from build123d import *

# Parameters (mm, degrees)
SKETCH1_R           = 8
SKETCH1_R_2         = 5
SKETCH1_R_3         = 3.5
BOSS_EXTRUDE1_DEPTH = 48.5
BOSS_EXTRUDE2_START = 18
SKETCH3_R           = 3.5
BOSS_EXTRUDE2_DEPTH = 18
FILLET1_DEPTH       = 19
CUT_EXTRUDE1_START  = -30.5
CUT_EXTRUDE1_DEPTH  = 30.5
BOSS_EXTRUDE3_DEPTH = 9.5


with BuildPart() as part:
    # Sketch1 → Boss-Extrude1 (new body)
    # profile 1 of 4: a face of its own
    with BuildSketch(Plane.XY):
        with BuildLine():
            Line((15, -14), (17.94787914, -14))
            ThreePointArc((17.94787914, -14), (20, -13.638155725), (21.804604798, -12.596266659))
            Line((21.804604798, -12.596266659), (33.266394429, -2.978683207))
            ThreePointArc((33.266394429, -2.978683207), (35.857071693, -1.449912319), (38.688110115, -0.433068885))
            Line((38.688110115, -0.433068885), (56, 4))
            ThreePointArc((56, 4), (51, 9), (56, 14))
            Line((56, 14), (15, 14))
            Line((15, 14), (15, -14))
        make_face()
    # profile 2 of 4: a face of its own
    with BuildSketch(Plane.XY):
        with BuildLine():
            Line((-8, -14), (15, -14))
            Line((15, -14), (15, 14))
            Line((15, 14), (-4, 14))
            ThreePointArc((-4, 14), (-11.071067812, 11.071067812), (-14, 4))
            Line((-14, 4), (-14, -8))
            ThreePointArc((-14, -8), (-12.242640687, -12.242640687), (-8, -14))
        make_face()
        Circle(SKETCH1_R, mode=Mode.SUBTRACT)
    # profile 3 of 4: a face of its own
    with BuildSketch(Plane.XY):
        with Locations((56, 9)):
            Circle(SKETCH1_R_2)
        with Locations((56, 9)):
            Circle(SKETCH1_R_3, mode=Mode.SUBTRACT)
    # profile 4 of 4: a face of its own
    with BuildSketch(Plane.XY):
        with Locations((56, 9)):
            Circle(SKETCH1_R_3)
    extrude(amount=-BOSS_EXTRUDE1_DEPTH)

    # Sketch3 → Boss-Extrude2 (add)
    with BuildSketch(Plane.XY.offset(BOSS_EXTRUDE2_START)):
        with BuildLine():
            Line((38.688110115, -0.433068885), (56, 4))
            ThreePointArc((56, 4), (51, 9), (56, 14))
            Line((56, 14), (15, 14))
            Line((15, 14), (15, -14))
            Line((15, -14), (17.94787914, -14))
            ThreePointArc((17.94787914, -14), (20, -13.638155725), (21.804604798, -12.596266659))
            Line((21.804604798, -12.596266659), (33.266394429, -2.978683207))
            ThreePointArc((33.266394429, -2.978683207), (35.857071693, -1.449912319), (38.688110115, -0.433068885))
        make_face()
        with Locations((56, 9)):
            Circle(SKETCH3_R)
    extrude(amount=-BOSS_EXTRUDE2_DEPTH)

    # Fillet1: read off the stored shape, not the designer's step
    # Fillet1 outline → Fillet1 (cut)
    with BuildSketch(Plane.XY):
        with BuildLine():
            ThreePointArc((56, 4), (55.277287525, 4.052507031), (54.569754044, 4.208925329))
            ThreePointArc((54.569754044, 4.208925329), (54.783881024, 3.915548669), (54.55835931, 3.630837966))
            Line((54.55835931, 3.630837966), (56, 4))
        make_face()
        with BuildLine():
            ThreePointArc((53.550510257, 14), (53.841896016, 13.771374643), (53.68916062, 13.433962264))
            ThreePointArc((53.68916062, 13.433962264), (54.810422621, 13.856429312), (56, 14))
            Line((56, 14), (53.550510257, 14))
        make_face()
    extrude(amount=FILLET1_DEPTH, mode=Mode.SUBTRACT)

    # Sketch6 → Cut-Extrude1 (cut)
    with BuildSketch(Plane(origin=(0, 0, -48.5), x_dir=(-1, 0, 0), z_dir=(0, 0, -1)).offset(CUT_EXTRUDE1_START)):
        with BuildLine():
            Line((-33.266394429, -2.978683207), (-21.804604798, -12.596266659))
            ThreePointArc((-21.804604798, -12.596266659), (-20, -13.638155725), (-17.94787914, -14))
            Line((-17.94787914, -14), (8, -14))
            ThreePointArc((8, -14), (12.242640687, -12.242640687), (14, -8))
            Line((14, -8), (14, 4))
            ThreePointArc((14, 4), (11.071067812, 11.071067812), (4, 14))
            Line((4, 14), (-56, 14))
            ThreePointArc((-56, 14), (-61, 9), (-56, 4))
            Line((-56, 4), (-38.688110115, -0.433068885))
            ThreePointArc((-38.688110115, -0.433068885), (-35.857071693, -1.449912319), (-33.266394429, -2.978683207))
        make_face()
    extrude(amount=CUT_EXTRUDE1_DEPTH, mode=Mode.SUBTRACT)

    # Sketch7 → Boss-Extrude3 (add)
    with BuildSketch(Plane(origin=(0, 0, -18), x_dir=(-1, 0, 0), z_dir=(0, 0, -1))):
        with BuildLine():
            Line((-33.266394429, -2.978683207), (-21.804604798, -12.596266659))
            ThreePointArc((-21.804604798, -12.596266659), (-20, -13.638155725), (-17.94787914, -14))
            Line((-17.94787914, -14), (8, -14))
            ThreePointArc((8, -14), (12.242640687, -12.242640687), (14, -8))
            Line((14, -8), (14, 4))
            ThreePointArc((14, 4), (11.071067812, 11.071067812), (4, 14))
            Line((4, 14), (-56, 14))
            ThreePointArc((-56, 14), (-61, 9), (-56, 4))
            Line((-56, 4), (-38.688110115, -0.433068885))
            ThreePointArc((-38.688110115, -0.433068885), (-35.857071693, -1.449912319), (-33.266394429, -2.978683207))
        make_face()
    extrude(amount=BOSS_EXTRUDE3_DEPTH)


solid = part.part
Read the model definition and answer for the solid it produces. Units are mm, in the model's axes. A direction names the side the tool comes from. Coordinates: 2 decimals unless noted, no trailing zeros. Loops run counter-clockwise (first coordinate to the right, second up) from the corner with the lowest first, then second, coordinate; pieces in that order, holes last.
Q1. The part is cut by section A-A on z = -12. Write down the section's boundary in (x, y), and give its area (3 significant figures).
Q2. The part is cut by section B-B on x = 0. Write down the section's boundary in (y, z), and give its area (3 significant figures).
Q3. Each of these flat-tipped pins is pushed along its axis until it touches: pin 1 Ø9 at (y, z) = (-5.5, 9.5) entering from -X; pin 2 Ø4 at (y, z) = (-6, -8) entering from +X; pin 3 Ø5 at (x, y) = (-0.5, -2) entering from +Z. Where does it stop, or does it pass through?
Q4. The part is cut by section C-C on z = -20.5. Write down the section's boundary in (x, y), and give its area (3 significant figures).
Q5. Which of the six approach directions +Z, -Z, +X, -X, +Y, -Y give full straight-line access (tool end or side, diameter ignored) to faces 4 (the face through (-12.196, -12.289, -13.558)), 5 (the face through (15, 0, 9)), 6 (the face through (52.503, 9.154, 9.126))?
Q6. The part is cut by section D-D on y = 0.75. Write down the section's boundary in (x, z).
Q7. Consider probe 1 along Y at (x, z) = (0, -4.75); probe 2 along Z at (x, y) = (3, -6.25); probe 3 along Z at (x, y) = (2, 12). Determine where each line is inside the solid, lowest interval first.
Q8. The mould has two halves that part along X. Classify faces 1 (the face through (56, 9, 18)), 2 (the face through (51.03, 8.44, 9.13)), 3 (the face through (27.616, -7.72, -4.432)): +X half, -X half, draft (parallel to the pull), parting line (faces both ways), or undercut.
Results below:
1. outline: (-14, -8) arc R6 ccw to (-8, -14) - (17.95, -14) arc R6 ccw to (21.8, -12.6) - (33.27, -2.98) arc R16 cw to (38.69, -0.43) - (56, 4) arc R5 ccw to (56, 14) - (-4, 14) arc R10 ccw to (-14, 4) - close; hole circle Ø16 at (0, 0)
1. area: 1,360 mm2
2. outline: (-14, -27.5) - (14, -27.5) - (14, 0) - (8, 0) - (8, -18) - (-8, -18) - (-8, 0) - (-14, 0) - close
2. area: 482 mm2
3. pin 1: stops at x = 15
3. pin 2: stops at x = 32.05
3. pin 3: stops at z = -18
4. outline: (-14, -8) arc R6 ccw to (-8, -14) - (17.95, -14) arc R6 ccw to (21.8, -12.6) - (33.27, -2.98) arc R16 cw to (38.69, -0.43) - (56, 4) arc R5 ccw to (56, 14) - (-4, 14) arc R10 ccw to (-14, 4) - close
4. area: 1,560 mm2
5. face 4: +Z, -Z, -X, -Y
5. face 5: +Z, -X, +Y, -Y
5. face 6: +Z
6. outline: (-14, -27.5) - (43.31, -27.5) - (43.31, 18) - (15, 18) - (15, 0) - (7.96, 0) - (7.96, -18) - (-7.96, -18) - (-7.96, 0) - (-14, 0) - close
7. probe 1: y = -14 to -8, 8 to 14
7. probe 2: z = -27.5 to -18
7. probe 3: z = -27.5 to 0
8. face 1: draft
8. face 2: undercut
8. face 3: +X half
